```python
from build123d import *

# Parameters (mm, degrees)
SKETCH2_R               = 3.75
BOSS_EXTRUDE1_DEPTH     = 3.75
SKETCH3_R               = 1.245
BOSS_EXTRUDE3_DEPTH     = 1.25
CUT_EXTRUDE2_DEPTH      = 8.288689869
CUT_EXTRUDE2_DEPTH_BACK = 8.288689869
SKETCH4_R               = 1.565
THREAD2_PITCH           = 1.5875


with BuildPart() as part:
    # Sketch2 → Boss-Extrude1 (new, symmetric)
    with BuildSketch(Plane.XY):
        Circle(SKETCH2_R)
    extrude(amount=BOSS_EXTRUDE1_DEPTH, both=True)

    # Sketch3 → Boss-Extrude3 (add)
    with BuildSketch(Plane.XY.offset(3.75)):
        Circle(SKETCH3_R)
    boss_extrude3 = extrude(amount=BOSS_EXTRUDE3_DEPTH)

    # Mirror1: Boss-Extrude3 across plane
    add(boss_extrude3.mirror(Plane.XY))

    # Sketch4 → Cut-Extrude2 (cut, two sides: drawn at the far end of the back side and taken through both)
    with BuildSketch(Plane(origin=(0, 0, 0), x_dir=(1, 0, 0), z_dir=(0, 1, 0)).offset(-CUT_EXTRUDE2_DEPTH_BACK)):
        with Locations(Location((0, 0, 0), (0, 0, 270))):
            Circle(SKETCH4_R)
    extrude(amount=CUT_EXTRUDE2_DEPTH + CUT_EXTRUDE2_DEPTH_BACK, mode=Mode.SUBTRACT)

    # Thread2: the profile of Thread Profile3 profile screwed along a right-hand helix of 3.401575 turns, 8 arcs to a turn; built about Z, then put on its axis
    thread2_z = Axis((0, 0, 0), (0, 0, 1))
    thread2_corners = [(1.5653, 0, -0.000173205), (1.5653, 0, 1.389235701), (0.705740423, 0, 0.892968748), (0.705740423, 0, 0.496093748)]
    with BuildLine(mode=Mode.PRIVATE) as thread2_profile:
        Line(thread2_corners[0], thread2_corners[1])
        Line(thread2_corners[1], thread2_corners[2])
        Line(thread2_corners[2], thread2_corners[3])
        Line(thread2_corners[3], thread2_corners[0])
    thread2_cap = Face(thread2_profile.wire())
    thread2_turn_angles = [0, 22.5, 45, 67.5, 90, 112.5, 135, 157.5, 180, 202.5, 225, 247.5, 270, 292.5, 315, 337.5, 360]
    thread2_turn_weights = [1, 0.9238795325112867, 1, 0.9238795325112867, 1, 0.9238795325112867, 1, 0.9238795325112867, 1, 0.9238795325112867, 1, 0.9238795325112867, 1, 0.9238795325112867, 1, 0.9238795325112867, 1]
    thread2_turn_rails = [Edge.make_bspline([Vector(p[0], p[1], 0).rotate(thread2_z, thread2_turn_angles[k]) / thread2_turn_weights[k] + Vector(0, 0, p[2] + THREAD2_PITCH * thread2_turn_angles[k] / 360) for k in range(17)], [0, 0, 0, 1, 1, 2, 2, 3, 3, 4, 4, 5, 5, 6, 6, 7, 7, 8, 8, 8], 2, thread2_turn_weights) for p in thread2_corners]
    thread2_turn_sides = [Face.make_surface_from_curves(thread2_turn_rails[p[0]], thread2_turn_rails[p[1]]) for p in [(0, 1), (1, 2), (2, 3), (3, 0)]]
    thread2_last_angles = [1080, 1102.5, 1125, 1147.5, 1170, 1192.5, 1215, 1219.783464567, 1224.566929134]
    thread2_last_weights = [1, 0.9238795325112867, 1, 0.9238795325112867, 1, 0.9238795325112867, 1, 0.9965169669882292, 1]
    thread2_last_rails = [Edge.make_bspline([Vector(p[0], p[1], 0).rotate(thread2_z, thread2_last_angles[k]) / thread2_last_weights[k] + Vector(0, 0, p[2] + THREAD2_PITCH * thread2_last_angles[k] / 360) for k in range(9)], [0, 0, 0, 1, 1, 2, 2, 3, 3, 4, 4, 4], 2, thread2_last_weights) for p in thread2_corners]
    thread2_last_sides = [Face.make_surface_from_curves(thread2_last_rails[p[0]], thread2_last_rails[p[1]]) for p in [(0, 1), (1, 2), (2, 3), (3, 0)]]
    thread2 = Plane(origin=(0, 3.4, 0), x_dir=(-1, 0, 0), z_dir=(0, -1, 0)) * Solid(Shell([*[p.moved(Location((0, 0, THREAD2_PITCH * i))) for i in range(3) for p in thread2_turn_sides], *thread2_last_sides, thread2_cap, thread2_cap.rotate(thread2_z, 1224.566929134).moved(Location((0, 0, THREAD2_PITCH * 1224.566929134 / 360)))]))
    add(thread2)


solid = part.part
```
Work out the finished part from the listing and answer in its coordinate system (mm). A direction names the side the tool comes from. Give positions to 0.01 mm unless a question says otherwise; leave off trailing zeros. Loops run counter-clockwise (first coordinate to the right, second up) from the corner with the lowest first, then second, coordinate; pieces in that order, holes last. Notation, with made-up numbers: (88.5, -1) - (129.5, -1) arc R25 cw to (129.5, 34) - close; hole circle Ø6 at (18.25, -29.75). An arc over 180 degrees is marked (long way). Use CSV: the item, a comma, the result in double quotes. Start each with the question number.
(1) Find section D-D, the plane z = 2.25. Determine the outline of the cut face in (x, y), plus the area to 3 significant figures.
(2) Find section C-C, the plane x = -1. Count the separate pieces of the cut face and the enclosed holes in it, plus the area to 3 significant figures.
(3) Find section A-A, the plane x = 3. Determine the outline of the cut face in (y, z).
(4) Determine the mould class of faces 1 (the face through (-1.2, 2.7, 0)), 2 (the face through (3.577, 1.126, 0.053)), 3 (the face through (0, 0, 5)) for opening direction X: released by +X, released by -X, zero draft, split by the parting line, or undercut.
(5) Find the intervals of material crossed by L1, parallel to Y at x = -1, z = -0.5; L2, parallel to Z at x = 0, y = -2.5 (3 decimals); L3, parallel to Z at x = 1.5, y = 2, in increasing order.
(6) A tool of negligible diameter and unlimited length cuts with its end or side. For faces 4 (the face through (-1, 1, -3.75)), 5 (the face through (-1, 1, 3.75)), 6 (the face through (0, 0, -5)), from which of +Z, -Z, +X, -X, +Y, -Y can it reach the whole face along a straight path? Write none if from no direction.
(7) Find section B-B, the plane z = 4.25. Determine the outline of the cut face in (x, y) (3 decimals).
(8) Each of these flat-tipped pins is pushed along its axis until it touches: pin 1 (4 mm diameter, centred on x = 0, z = 0, fed in from +Y); pin 2 (2 mm diameter, centred on x = 0, y = 2.5, fed in from -Z); pin 3 (1.5 mm diameter, centred on x = 1.5, y = -2.5, fed in from +Z); pin 4 (2.5 mm diameter, centred on x = 0, z = 0, fed in from +Y). Where does it stop, or does it pass through?
Results found:
1,outline,"circle Ø7.5 at (0, 0)"
1,area,"44.2 mm^2"
2,separate pieces,"1"
2,enclosed holes,"2"
2,area,"48.7 mm^2"
3,outline,"(-2.25, -3.75) - (2.25, -3.75) - (2.25, 3.75) - (-2.25, 3.75) - close"
4,face 1,"undercut"
4,face 2,"split by the parting line"
4,face 3,"zero draft"
5,L1,"-2.61 to -1.74, -1.02 to -0.15, 0.56 to 1.44, 2.15 to 3.02"
5,L2,"-3.75 to -0.706, 1.565 to 3.75"
5,L3,"-3.75 to 3.75"
6,face 4,"-Z"
6,face 5,"+Z"
6,face 6,"-Z, +X, -X, +Y, -Y"
7,outline,"circle Ø2.49 at (0, 0)"
8,pin 1,"y = 3.75"
8,pin 2,"z = -3.75"
8,pin 3,"z = 3.75"
8,pin 4,"y = 3.22"
